from build123d import *

# Parameters (mm, degrees)
F0_R      = 59.055
F1_DEPTH  = 5.08
F3_DEPTH  = 5.08
F4_COUNT  = 20
F5_R      = 50.8
F6_DEPTH  = 5.081
F7_DEPTH  = 5.081
F9_DEPTH  = 5.08
F10_COUNT = 3
F11_R     = 3.302
F12_DEPTH = 5.081


with BuildPart() as f1:
    # F0 (on Top) → F1 (new body)
    with BuildSketch(Plane.XY):
        Circle(F0_R)
    extrude(amount=F1_DEPTH)

    # F4: F3 ×20 about axis
    f4_axis = Axis((0, 0, 5.08), (0, 0, 1))


with BuildPart() as f3:
    # F2 (on face) → F3 (new body, through all)
    with BuildSketch(Plane.XY.offset(5.08)):
        with BuildLine():
            Line((-6.7921649906, 58.5710500385), (1.5174926213, 58.9440295875))
            ThreePointArc((1.5174926213, 58.9440295875), (-0.0730129244, 63.6408133417), (-3.035026947, 67.6177416104))
            ThreePointArc((-3.035026947, 67.6177416104), (-5.6288384248, 63.3914397349), (-6.7921649906, 58.5710500385))
        make_face()
    extrude(amount=-F3_DEPTH)


with BuildPart() as f1_1:
    add(f1.part)
    for i in range(1, F4_COUNT):
        add(f3.part.rotate(f4_axis, i * 360 / F4_COUNT))

    # F5 (on face) → F6 (cut, through all)
    with BuildSketch(Plane.XY.offset(5.08)):
        Circle(F5_R)
    extrude(amount=-F6_DEPTH, mode=Mode.SUBTRACT)

    # F5 (on face) → F7 (cut, through all)
    with BuildSketch(Plane.XY.offset(5.08)):
        Circle(F5_R)
    extrude(amount=-F7_DEPTH, mode=Mode.SUBTRACT)



with BuildPart() as f9:
    # F8 (on face) → F9 (new body, through all)
    with BuildSketch(Plane.XY.offset(5.08)):
        with BuildLine():
            Line((-8.8213274255, 50.028233853), (-1.1026659282, 6.2535292316))
            ThreePointArc((-1.1026659282, 6.2535292316), (0, -6.35), (1.1026659282, 6.2535292316))
            Line((1.1026659282, 6.2535292316), (8.8213274255, 50.028233853))
            ThreePointArc((8.8213274255, 50.028233853), (0, 50.8), (-8.8213274255, 50.028233853))
        make_face()
    extrude(amount=-F9_DEPTH)


with BuildPart() as f1_2:
    add(f1_1.part)

    add(f3.part)  # F10 merges F3

    add(f9.part)  # F10 merges F9
    # F10: F9 ×3 about axis
    f10_axis = Axis((0, 0, 5.08), (0, 0, 1))
    for i in range(1, F10_COUNT):
        add(f9.part.rotate(f10_axis, i * 360 / F10_COUNT))

    # F11 (on face) → F12 (cut, through all)
    with BuildSketch(Plane.XY.offset(5.08)):
        Circle(F11_R)
    extrude(amount=-F12_DEPTH, mode=Mode.SUBTRACT)


solid = f1_2.part
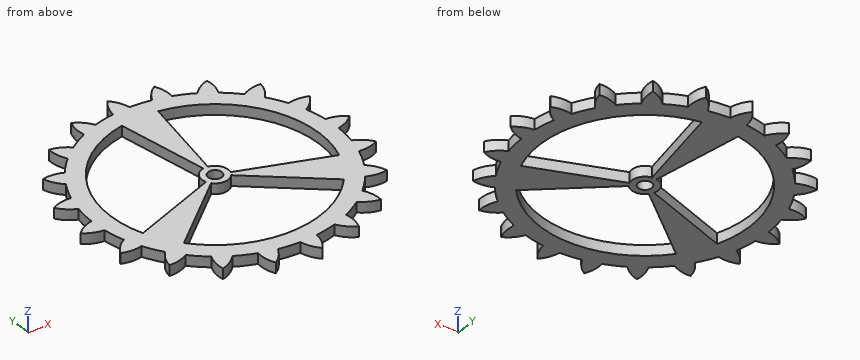
Could you check a few things on this model? Use its own coordinates, in mm. Coordinates: 2 decimals unless noted, no trailing zeros. One line per question, with ' | ' between items.
Q1. If I drill on L1, parallel to Y at x = 0, z = 3.35; L2, parallel to Y at x = -25.5, z = 0.8; L3, parallel to X at y = -42.5, z = 0.4, over which ranges is the centre line in solid material (lowest first)?
Return value:
L1: -63.5 to -50.8, -6.35 to -3.3, 3.3 to 63.5 | L2: -53.27 to -43.94, -21.4 to -9.28, 43.94 to 53.27 | L3: -41 to -27.83, 27.83 to 41
Q2. Imagine slicing it at A-A on z = 1.3. State how many separate pieces and enclosed holes the cut face has, and give its area (3 significant figures).
Return value:
separate pieces: 1 | enclosed holes: 4 | area: 5,180 mm²
Q3. I'm going to push flat-ended pins straight in: P1, Ø8, axis at x = -38, y = -47, coming from the +Z side; P2, Ø1.5, axis at y = -36, z = 0.5, coming from the +X side; P3, Ø1, axis at x = 51, z = 1, coming from the -Y side. Where does each tip first touch, or does it pass through?
Return value:
P1: z = 5.08 | P2: x = 56.35 | P3: y = -37.34
